Can you work these out from the model? Positions are in its coordinate system, mm. A direction names the side the tool comes from. Give positions to 0.01 mm unless a question says otherwise; leave off trailing zeros. Write each loop counter-clockwise with the first axis right and the second up, starting at its lowest first coordinate (ties: lowest second). Pieces come first, ordered by that corner, then holes.
from build123d import *

# Parameters (mm, degrees)
SKETCH1_R           = 9
SKETCH1_R_2         = 5
BOSS_EXTRUDE1_DEPTH = 6.26
BOSS_EXTRUDE2_DEPTH = 6.26
SKETCH2_R           = 7
CUT_EXTRUDE1_DEPTH  = 4.41
SKETCH4_W           = 36.26
SKETCH4_H           = 18
BOSS_EXTRUDE3_DEPTH = 4
SKETCH5_R           = 5
CUT_EXTRUDE2_DEPTH  = 5
BOSS_EXTRUDE4_DEPTH = 50


with BuildPart() as part:
    # Sketch1 → Boss-Extrude1 (new body)
    with BuildSketch(Plane(origin=(0, 0, 0), x_dir=(0, 0, -1), z_dir=(1, 0, 0))):
        Circle(SKETCH1_R)
        Circle(SKETCH1_R_2, mode=Mode.SUBTRACT)
    extrude(amount=BOSS_EXTRUDE1_DEPTH)

    # Sketch3 → Boss-Extrude2 (add)
    with BuildSketch(Plane.ZY):
        with BuildLine():
            Line((-9, 0), (-9, -30))
            Line((-9, -30), (9, -30))
            Line((9, -30), (9, 0))
            Line((9, 0), (5, 0))
            ThreePointArc((5, 0), (0, -5), (-5, 0))
            Line((-5, 0), (-9, 0))
        make_face()
    extrude(amount=-BOSS_EXTRUDE2_DEPTH)

    # Sketch2 → Cut-Extrude1 (cut)
    with BuildSketch(Plane(origin=(6.26, 0, 0), x_dir=(0, 0, -1), z_dir=(1, 0, 0))):
        Circle(SKETCH2_R)
    extrude(amount=-CUT_EXTRUDE1_DEPTH, mode=Mode.SUBTRACT)

    # Sketch4 → Boss-Extrude3 (add)
    with BuildSketch(Plane.XZ.offset(30)):
        with Locations((-11.87, 0)):
            Rectangle(SKETCH4_W, SKETCH4_H)
    extrude(amount=BOSS_EXTRUDE3_DEPTH)

    # Mirror2: part across plane


with BuildPart() as part_1:
    add(part.part)
    add(part.part.mirror(Plane(origin=(-30, -34, 9), x_dir=(0, 0, 1), z_dir=(1, 0, 0))))

    # Sketch5 → Cut-Extrude2 (cut, through all)
    with BuildSketch(Plane(origin=(0, -30, 0), x_dir=(1, 0, 0), z_dir=(0, 1, 0))):
        with Locations((-30, 0)):
            Circle(SKETCH5_R)
    extrude(amount=-CUT_EXTRUDE2_DEPTH, mode=Mode.SUBTRACT)

    # Sketch6 → Boss-Extrude4 (add)
    with BuildSketch(Plane.XZ.offset(34)):
        with BuildLine():
            ThreePointArc((1.184711928, 18.501387568), (6.224007517, -1.615202581), (-0.585698563, -21.203454222))
            ThreePointArc((-0.585698563, -21.203454222), (-7.565532493, -22.335672537), (-8.697750807, -15.355838607))
            ThreePointArc((-8.697750807, -15.355838607), (-3.76606626, -1.169752338), (-7.415594726, 13.39896408))
            ThreePointArc((-7.415594726, 13.39896408), (-5.666653143, 20.250329151), (1.184711928, 18.501387568))
        make_face()
        with BuildLine():
            ThreePointArc((-61.638666525, 17.713903593), (-66.200917241, -2.069103891), (-59.414301437, -21.203454222))
            ThreePointArc((-59.414301437, -21.203454222), (-52.434467507, -22.335672537), (-51.302249193, -15.355838607))
            ThreePointArc((-51.302249193, -15.355838607), (-56.217211438, -1.498474026), (-52.913165553, 12.828657153))
            ThreePointArc((-52.913165553, 12.828657153), (-54.833292819, 19.634030859), (-61.638666525, 17.713903593))
        make_face()
    extrude(amount=BOSS_EXTRUDE4_DEPTH)


solid = part_1.part
(1) Imagine slicing it at A-A, the plane y = -15. Write out the boundary of the cut face in (x, z).
Returned:
outline: (-66.26, -9) - (-60, -9) - (-60, 9) - (-66.26, 9) - close; (0, -9) - (6.26, -9) - (6.26, 9) - (0, 9) - close
(2) Imagine slicing it at C-C, the plane z = 3.5. Give the number of separate pieces and of enclosed holes in the cut face, plus the area to 3 significant figures.
Returned:
separate pieces: 4
enclosed holes: 0
area: 1,610 mm2
(3) Imagine slicing it at D-D, the plane x = -15.5. Write out the boundary of the cut face in (y, z), plus the area to 3 significant figures.
Returned:
outline: (-34, -9) - (-30, -9) - (-30, 9) - (-34, 9) - close
area: 72.0 mm2
(4) If I drill on L1, parallel to Y at x = 1.5, z = 0; L2, parallel to X at y = -20, z = 3; L3, parallel to Z at x = -30, y = -32, over which ranges is the centre line in solid material (lowest first)?
Returned:
L1: y = -84 to -5, 5 to 9
L2: x = -66.26 to -60, 0 to 6.26
L3: z = -9 to -5, 5 to 9
(5) Will these pins go through, and if not, where does the flat tip stop? P1, Ø17, axis at x = -14.5, y = -24, coming from the -Z side; P2, Ø12.5, axis at y = 0, z = 0, coming from the +X side; P3, Ø5.5, axis at x = -15, z = -3.5, coming from the +Y side; P4, Ø11, axis at y = 3, z = 1.5, coming from the -X side.
Returned:
P1: stops at z = -9
P2: stops at x = 1.85
P3: stops at y = -30
P4: stops at x = -66.26
(6) If we mould it in two halves opening along X, with no side actions, what happens to faces 4 (the face through (6.26, -17, 0)), 5 (the face through (-52.524, -58.65, -22.399)), 6 (the face through (4.086, -2.681, -6.466))? For each: +X half, -X half, draft (parallel to the pull), parting line (faces both ways), or undercut.
Returned:
face 4: +X half
face 5: undercut
face 6: draft
(7) Imagine slicing it at B-B, the plane x = -30. Write out the boundary of the cut face in (y, z).
Returned:
outline: (-34, -9) - (-30, -9) - (-30, -5) - (-34, -5) - close; (-34, 5) - (-30, 5) - (-30, 9) - (-34, 9) - close
(8) For faces 1 (the face through (-1, -34, 15)), 2 (the face through (6.236, -58.65, -1.321)), 3 (the face through (-61.85, 5, 2)), which set-ups out of +Z, -Z, +X, -X, +Y, -Y let a thin tool reach every point of the face, with its end or its side?
Returned:
face 1: +Z, +X, -X, +Y
face 2: +X, -Y
face 3: -X
